```python
from build123d import *

# Parameters (mm, degrees)
PAD_DEPTH          = 70
SKETCH002_W        = 20
SKETCH002_H        = 20
PAD001_DEPTH       = 2
SKETCH003_R        = 1
POCKET_DEPTH       = 5
POLARPATTERN_COUNT = 4


with BuildPart() as pad:
    # Sketch001 → Pad (new body)
    with BuildSketch(Plane.XY):
        with BuildLine():
            Line((-5, 4), (-5, 5))
            Line((-5, 5), (5, 5))
            Line((5, 5), (5, 4))
            Line((5, 4), (1.5, 4))
            ThreePointArc((1.5, 4), (0.651472, 3.648528), (0.3, 2.8))
            Line((0.3, 2.8), (0.3, -2.8))
            ThreePointArc((0.3, -2.8), (0.651472, -3.648528), (1.5, -4))
            Line((1.5, -4), (5, -4))
            Line((5, -4), (5, -5))
            Line((5, -5), (-5, -5))
            Line((-5, -5), (-5, -4))
            Line((-5, -4), (-1.5, -4))
            ThreePointArc((-1.5, -4), (-0.651472, -3.648528), (-0.3, -2.8))
            Line((-0.3, -2.8), (-0.3, 2.8))
            ThreePointArc((-0.3, 2.8), (-0.651472, 3.648528), (-1.5, 4))
            Line((-1.5, 4), (-5, 4))
        make_face()
    extrude(amount=PAD_DEPTH)


with BuildPart() as fusion:
    # Sketch002 → Pad001 (new body)
    with BuildSketch(Plane.XY):
        Rectangle(SKETCH002_W, SKETCH002_H)
    extrude(amount=PAD001_DEPTH)

    # Sketch003 → Pocket (cut)
    with BuildSketch(Plane.XY.offset(2)):
        with Locations((-7, 7)):
            Circle(SKETCH003_R)
    pocket = extrude(amount=-POCKET_DEPTH, mode=Mode.SUBTRACT)

    # PolarPattern: Pocket ×4 about axis
    polarpattern_axis = Axis((0, 0, 2), (0, 0, 1))
    for i in range(1, POLARPATTERN_COUNT):
        add(pocket.rotate(polarpattern_axis, i * 360 / POLARPATTERN_COUNT), mode=Mode.SUBTRACT)

    # Fusion: union Pad
    add(pad.part)


solid = fusion.part
```
For this review, take the finished solid that the model builds, in its own axes (mm). A direction names the side the tool comes from. Give positions to 0.01 mm unless a question says otherwise; leave off trailing zeros. Loops run counter-clockwise (first coordinate to the right, second up) from the corner with the lowest first, then second, coordinate; pieces in that order, holes last. Notation, with made-up numbers: M -31,31 L -14,31 A19 cw -14,42 Z; hole C 24.5,22 d3. An arc over 180 degrees is marked long. One line per item, written item: value. Start each with the question number.
Q1. For L1, parallel to X at y = -7, z = 0.7; L2, parallel to Y at x = -3, z = 48, list the stretches that pass through material, from the lowest coordinate up.
Q2. Add section A-A (x = 7). Give the boundary of the cut face in (y, z).
Q3. Add section C-C (z = 48). Give the boundary of the cut face in (x, y), and give its area (3 significant figures).
Q4. Clearance check with flat-ended pins moving along their axes: pin 1 Ø1.2 at (x, y) = (7, 7) entering from -Z; pin 2 Ø1 at (x, z) = (-4, 19.5) entering from -Y; pin 3 Ø3 at (x, z) = (-0.5, 32) entering from +Y; pin 4 Ø1.7 at (y, z) = (0.5, 40) entering from +X. State where each tip first meets the part, or that it passes through.
Q5. Machinability: for faces 4 (the face through (-3, -4, 36)), 5 (the face through (8, 7, 1)), 6 (the face through (0, -5, 36)), 7 (the face through (0.661, 3.658, 35.524)), which of the approach directions +Z, -Z, +X, -X, +Y, -Y give a long, thin tool a straight path to every point of the face, cutting with its end or side? Answer none if there is none.
Q6. Add section D-D (x = 2.5). Give the boundary of the cut face in (y, z), and give its area (3 significant figures).
Q7. Draft analysis for pull direction X (two halves, no side actions). For faces 1 (the face through (7, -8, 1)), 2 (the face through (-3, 4, 36)), 3 (the face through (-0.661, -3.658, 35.524)), state which applies: released by +X, released by -X, zero draft, split by the parting line, or undercut.
Reply:
1. L1: -10 to -8, -6 to 6, 8 to 10
1. L2: -5 to -4, 4 to 5
2. outline: M -10,0 L -8,0 L -8,2 L -10,2 Z; M -6,0 L 6,0 L 6,2 L -6,2 Z; M 8,0 L 10,0 L 10,2 L 8,2 Z
3. outline: M -5,-5 L 5,-5 L 5,-4 L 1.5,-4 A1.2 cw 0.3,-2.8 L 0.3,2.8 A1.2 cw 1.5,4 L 5,4 L 5,5 L -5,5 L -5,4 L -1.5,4 A1.2 cw -0.3,2.8 L -0.3,-2.8 A1.2 cw -1.5,-4 L -5,-4 Z
3. area: 26.0 mm²
4. pin 1: through
4. pin 2: y = -5
4. pin 3: y = 5
4. pin 4: x = 0.3
5. face 4: +Z, -X
5. face 5: +Z, -Z
5. face 6: +Z, +X, -X, -Y
5. face 7: +Z, +X
6. outline: M -10,0 L 10,0 L 10,2 L 5,2 L 5,70 L 4,70 L 4,2 L -4,2 L -4,70 L -5,70 L -5,2 L -10,2 Z
6. area: 176 mm²
7. face 1: undercut
7. face 2: zero draft
7. face 3: released by -X
